```python
from build123d import *

# Parameters (mm, degrees)
F0_W       = 228.6
F0_H       = 279.4
F1_DEPTH   = 25.4
F2_W       = 19.05
F2_H       = 279.4
F3_DEPTH   = 12.7
F4_W       = 19.05
F4_H       = 279.4
F5_DEPTH   = 12.7
F6_W       = 190.5
F6_H       = 19.05
F7_DEPTH   = 12.7
F8_W       = 12.7
F8_H       = 63.5
F9_DEPTH   = 57.15
F10_W      = 12.7
F10_H      = 63.5
F11_DEPTH  = 57.15
F13_DEPTH  = 12.7
F14_W      = 342.9
F14_H      = 12.7
F15_DEPTH  = 12.7
F16_W      = 25.4
F16_H      = 12.7
F17_W      = 25.4
F17_H      = 12.7
F18_W      = 25.4
F18_H      = 12.7
F19_DEPTH  = 12.7
F19_FACE_W = 12.7
F19_FACE_H = 12.7
F20_DEPTH  = 304.8


with BuildPart() as f1:
    # F0 (on Front) → F1 (new body)
    with BuildSketch(Plane.XZ):
        with Locations((114.3, 139.7)):
            Rectangle(F0_W, F0_H)
    extrude(amount=F1_DEPTH)

    # F2 (on face) → F3 (cut)
    with BuildSketch(Plane.XZ.offset(25.4)):
        with Locations((219.075, 139.7)):
            Rectangle(F2_W, F2_H)
    extrude(amount=-F3_DEPTH, mode=Mode.SUBTRACT)

    # F4 (on face) → F5 (cut)
    with BuildSketch(Plane.XZ.offset(25.4)):
        with Locations((9.525, 139.7)):
            Rectangle(F4_W, F4_H)
    extrude(amount=-F5_DEPTH, mode=Mode.SUBTRACT)

    # F6 (on face) → F7 (cut)
    with BuildSketch(Plane.XZ.offset(25.4)):
        with Locations((114.3, 269.875)):
            Rectangle(F6_W, F6_H)
    extrude(amount=-F7_DEPTH, mode=Mode.SUBTRACT)

    # F8 (on face) → F9 (join)
    with BuildSketch(Plane.YZ.offset(228.6)):
        with Locations((-6.35, 31.75)):
            Rectangle(F8_W, F8_H)
    extrude(amount=F9_DEPTH)

    # F10 (on face) → F11 (join)
    with BuildSketch(Plane(origin=(0, 0, 0), x_dir=(0, -1, 0), z_dir=(-1, 0, 0))):
        with Locations((6.35, 31.75)):
            Rectangle(F10_W, F10_H)
    extrude(amount=F11_DEPTH)

    # F12 (on face) → F13 (join)
    with BuildSketch(Plane.XZ.offset(12.7)):
        Polygon((0, 63.5), (-57.15, 63.5), (-57.15, 0), (19.05, 0), (19.05, 63.5), align=None)
        Polygon((285.75, 63.5), (228.6, 63.5), (209.55, 63.5), (209.55, 0), (285.75, 0), align=None)
    extrude(amount=F13_DEPTH)

    # F14 (on face) → F15 (cut)
    with BuildSketch(Plane.XZ.offset(25.4)):
        Polygon((-57.15, 63.5), (-57.15, 50.8), (285.75, 50.8), (285.75, 63.5), (209.55, 63.5), (19.05, 63.5), align=None)
        with Locations((114.3, 31.75)):
            Rectangle(F14_W, F14_H)
        with Locations((114.3, 6.35)):
            Rectangle(F14_W, F14_H)
    extrude(amount=-F15_DEPTH, mode=Mode.SUBTRACT)

    # F16 (on face) + F17 (on face) + F18 (on face) → F19 (join)
    with BuildSketch(Plane.XZ.offset(12.7)):
        with Locations((-44.45, 57.15)):
            Rectangle(F16_W, F16_H)
        with Locations((273.05, 57.15)):
            Rectangle(F16_W, F16_H)
    with BuildSketch(Plane.XZ.offset(12.7)):
        with Locations((-44.45, 31.75)):
            Rectangle(F17_W, F17_H)
        with Locations((273.05, 31.75)):
            Rectangle(F17_W, F17_H)
    with BuildSketch(Plane.XZ.offset(12.7)):
        with Locations((-44.45, 6.35)):
            Rectangle(F18_W, F18_H)
        with Locations((273.05, 6.35)):
            Rectangle(F18_W, F18_H)
    extrude(amount=F19_DEPTH)

    # F19_face (on face) → F20 (join)
    with BuildSketch(Plane(origin=(-31.75, -19.05, 57.15), x_dir=(0, 1, 0), z_dir=(1, 0, 0))):
        Rectangle(F19_FACE_W, F19_FACE_H)
    extrude(amount=F20_DEPTH)


solid = f1.part
```
Could you check a few things on this model? Use its own coordinates, in mm. A direction names the side the tool comes from. Coordinates: 2 decimals unless noted, no trailing zeros. Write each loop counter-clockwise with the first axis right and the second up, starting at its lowest first coordinate (ties: lowest second). Pieces come first, ordered by that corner, then holes. Notation, with made-up numbers: (-8, 71) -> (24, 71) arc R30 ccw to (24, 107) -> close; hole circle Ø3 at (3.25, 40.5). An arc over 180 degrees is marked (long way). One line per question, with ' | ' between items. Start each with the question number.
1. Please list where these lines run through material, in increasing order: line 1 along Z through (x, y) = (31, -19.5); line 2 along Y through (x, z) = (227, 157); line 3 along X through (y, z) = (-23, 64).
2. For faces 1 (the face through (228.6, -6, 170)), 2 (the face through (-31.75, -19, 32)), 3 (the face through (-31.75, -19, 6)), 4 (the face through (0, -6, 170)), which set-ups out of +Z, -Z, +X, -X, +Y, -Y let a thin tool reach every point of the face, with its end or its side?
3. Thinking about a two-plate mould opening in X: for faces 5 (the face through (112, -12.7, 32)), 6 (the face through (209.55, -19, 161)), 7 (the face through (113, -6, 279.4)), which applies, pulls with the +X half, pulls with the -X half, needs draft (parallel to the pull), parting line crosses it, or undercut?
4. If we section it at A-A (y = -20.25): Please give me the cut outline in (x, z), and give its area (3 significant figures).
5. If we section it at B-B (x = 105): Please give me the cut outline in (y, z).
6. Will these pins go through, and if not, where does the flat tip stop? P1, Ø5, axis at x = 215, z = 217.5, coming from the -Y side; P2, Ø4, axis at y = -20, z = 177.5, coming from the -X side; P3, Ø1, axis at x = 23.5, y = -15.5, coming from the -Z side.
7. If we section it at C-C (z = 155.5): Please give me the cut outline in (x, y).
8. If we section it at D-D (x = -36): Please give me the cut outline in (y, z), and give its area (3 significant figures).
Return value:
1) line 1: z = 12.7 to 25.4, 38.1 to 260.35 | line 2: y = -12.7 to 0 | line 3: x = 19.05 to 209.55
2) face 1: +Z, +X, +Y, -Y | face 2: -Y | face 3: -Z, -Y | face 4: +Z, -X, +Y, -Y
3) face 5: undercut | face 6: pulls with the +X half | face 7: needs draft
4) outline: (-57.15, 0) -> (-31.75, 0) -> (-31.75, 12.7) -> (260.35, 12.7) -> (260.35, 0) -> (285.75, 0) -> (285.75, 63.5) -> (209.55, 63.5) -> (209.55, 260.35) -> (19.05, 260.35) -> (19.05, 63.5) -> (-57.15, 63.5) -> close; hole (-31.75, 25.4) -> (260.35, 25.4) -> (260.35, 38.1) -> (-31.75, 38.1) -> close | area: 51,900 mm²
5) outline: (-25.4, 12.7) -> (-12.7, 12.7) -> (-12.7, 0) -> (0, 0) -> (0, 279.4) -> (-12.7, 279.4) -> (-12.7, 260.35) -> (-25.4, 260.35) -> (-25.4, 38.1) -> (-12.7, 38.1) -> (-12.7, 25.4) -> (-25.4, 25.4) -> close
6) P1: stops at y = -12.7 | P2: stops at x = 19.05 | P3: stops at z = 12.7
7) outline: (0, -12.7) -> (19.05, -12.7) -> (19.05, -25.4) -> (209.55, -25.4) -> (209.55, -12.7) -> (228.6, -12.7) -> (228.6, 0) -> (0, 0) -> close
8) outline: (-25.4, 0) -> (0, 0) -> (0, 63.5) -> (-25.4, 63.5) -> close | area: 1,610 mm²
